from build123d import *

# Parameters (mm, degrees)
SKETCH_1_R               = 80
SKETCH_1_R_2             = 10.5
EXTRUDE_1_DEPTH          = 80
SKETCH_2_R               = 20
CUT_EXTRUDE_1_DEPTH      = 10
SKETCH_3_R               = 20
CUT_EXTRUDE_2_DEPTH      = 20
CUT_EXTRUDE_3_DEPTH      = 70
PATTERN_CIRCULAR_1_COUNT = 18
SKETCH_6_R               = 35
CUT_EXTRUDE_4_DEPTH      = 10
SKETCH_7_R               = 40
SKETCH_7_R_2             = 20
EXTRUDE_2_DEPTH          = 10
CUT_EXTRUDE_5_DEPTH      = 10


with BuildPart() as part:
    # 草图1 → 凸台-拉伸1 (new body)
    with BuildSketch(Plane.XY):
        Circle(SKETCH_1_R)
        Circle(SKETCH_1_R_2, mode=Mode.SUBTRACT)
    extrude(amount=EXTRUDE_1_DEPTH)

    # 草图2 → 切除-拉伸1 (cut)
    with BuildSketch(Plane.XY.offset(80)):
        Circle(SKETCH_2_R)
    extrude(amount=-CUT_EXTRUDE_1_DEPTH, mode=Mode.SUBTRACT)

    # 草图3 → 切除-拉伸2 (cut)
    with BuildSketch(Plane(origin=(0, 0, 0), x_dir=(-1, 0, 0), z_dir=(0, 0, -1))):
        Circle(SKETCH_3_R)
    extrude(amount=-CUT_EXTRUDE_2_DEPTH, mode=Mode.SUBTRACT)

    # 草图4 → 切除-拉伸3 (cut)
    with BuildSketch(Plane(origin=(0, 0, 5), x_dir=(-1, 0, 0), z_dir=(0, 0, -1))):
        with BuildLine():
            Line((-6.649138428, 76), (-6.97245942, 79.695575847))
            ThreePointArc((-6.97245942, 79.695575847), (0, 80), (6.97245942, 79.695575847))
            Line((6.97245942, 79.695575847), (6.649138428, 76))
            Line((6.649138428, 76), (-6.649138428, 76))
        make_face()
    cut_extrude_3 = extrude(amount=-CUT_EXTRUDE_3_DEPTH, mode=Mode.SUBTRACT)

    # 阵列(圆周)1: 切除-拉伸3 ×18 about axis
    pattern_circular_1_axis = Axis((0, 0, 0), (0, 0, 1))
    for i in range(1, PATTERN_CIRCULAR_1_COUNT):
        add(cut_extrude_3.rotate(pattern_circular_1_axis, i * 360 / PATTERN_CIRCULAR_1_COUNT), mode=Mode.SUBTRACT)

    # 草图6 → 切除-拉伸4 (cut)
    with BuildSketch(Plane(origin=(0, 0, 0), x_dir=(-1, 0, 0), z_dir=(0, 0, -1))):
        Circle(SKETCH_6_R)
    extrude(amount=-CUT_EXTRUDE_4_DEPTH, mode=Mode.SUBTRACT)

    # 草图7 → 凸台-拉伸2 (add)
    with BuildSketch(Plane.XY.offset(80)):
        Circle(SKETCH_7_R)
        Circle(SKETCH_7_R_2, mode=Mode.SUBTRACT)
    extrude(amount=EXTRUDE_2_DEPTH)

    # 草图8 → 切除-拉伸5 (cut)
    with BuildSketch(Plane.XY.offset(90)):
        Polygon((34.641016151, 0), (17.320508076, 30), (-17.320508076, 30), (-34.641016151, 0), (-17.320508076, -30), (17.320508076, -30), align=None)
    extrude(amount=-CUT_EXTRUDE_5_DEPTH, mode=Mode.SUBTRACT)


solid = part.part
Geometry: final body of the model. Coordinates: model frame, mm. A direction names the side the tool comes from. Give positions to 0.01 mm unless a question says otherwise; leave off trailing zeros. Loops run counter-clockwise (first coordinate to the right, second up) from the corner with the lowest first, then second, coordinate; pieces in that order, holes last. Notation, with made-up numbers: M 61.5,-32 L 73.5,-32 A12 ccw 73.5,-24 Z; hole C 45.25,33 d4. An arc over 180 degrees is marked long. Put each result on its own line as item: value. Start each with the question number.
1) Cut plane A-A (y = -27). Output: boundary loops of the cut face in (x, z), then the cut area to 3 significant figures.
2) Access query for faces 5 (the flat face through (-48.92, 58.16, 39.51)), 6 (the flat face through (-15, -15, 10)), 7 (the flat face through (0, 78, 5)), 8 (the flat face through (9, -9, 70)). Directions: +Z, -Z, +X, -X, +Y, -Y. A direction counts if a zero-diameter tool reaches every point of the face in a straight line with its end or side. Return the directions, or none.
3) Cut plane B-B (y = -60.5). Output: boundary loops of the cut face in (x, z), then the cut area to 3 significant figures.
4) Ray query, line 1 along Y through (x, z) = (0, 2); line 2 along Y through (x, z) = (0, 72.25); line 3 along Z through (x, y) = (-50.5, 32.5). Return the intervals inside material, ascending.
5) Contact query for flat-ended pins moving along their axis: pin 1 (3 mm diameter, centred on x = -3.5, y = -77, fed in from +Z); pin 2 (12 mm diameter, centred on x = -8, y = 7, fed in from -Z); pin 3 (2 mm diameter, centred on y = 31, z = 40.5, fed in from -X). Output: stop coordinate, or through.
6) Pull-direction query (Z, two-part tool) for faces 1 (the flat face through (-77, 13, 5)), 2 (the flat face through (-68, 39, 75)), 3 (the cylindrical face through (-4.336, -19.524, 74.93)), 4 (the flat face through (-27, -15, 90)); classes: pulls with the +Z half, pulls with the -Z half, needs draft (parallel to the pull), parting line crosses it, or undercut.
Verdict:
1. outline: M -75.31,0 L -22.27,0 L -22.27,10 L 22.27,10 L 22.27,0 L 75.31,0 L 75.31,80 L 29.51,80 L 29.51,90 L 19.05,90 L 19.05,80 L -19.05,80 L -19.05,90 L -29.51,90 L -29.51,80 L -75.31,80 Z
1. area: 11,800 mm2
2. face 5: none
2. face 6: -Z
2. face 7: +Y
2. face 8: +Z
3. outline: M -52.34,0 L 52.34,0 L 52.34,5 L 46.13,5 L 46.13,75 L 52.34,75 L 52.34,80 L -52.34,80 L -52.34,75 L -46.13,75 L -46.13,5 L -52.34,5 Z
3. area: 7,510 mm2
4. line 1: -80 to -35, 35 to 80
4. line 2: -76 to -20, 20 to 76
4. line 3: 0 to 80
5. pin 1: z = 80
5. pin 2: z = 20
5. pin 3: x = -74.16
6. face 1: undercut
6. face 2: undercut
6. face 3: needs draft
6. face 4: pulls with the +Z half
